```python
from build123d import *

# Parameters (mm, degrees)
F2_DEPTH = 1.778
F3_D     = 3.302
F4_W     = 6.35
F4_H     = 14.4874919379
F4_W_2   = 9.525
F4_W_3   = 11.43
F4_H_2   = 7.62
F4_W_4   = 1.905
F5_DEPTH = 7.62


with BuildPart() as f2:
    # F0 (on Front) → F2 (new body)
    with BuildSketch(Plane.XZ):
        Polygon((-50.8, 24.0124919379), (-50.8, -29.3275080621), (-36.83, -29.3275080621), (0, -29.3275080621), (15.24, -29.3275080621), (15.24, -26.7875080621), (17.235215947, -25.2156577751), (17.235215947, 7.5503422249), (15.24, 9.122192512), (15.24, 20.552192512), (13.716, 24.0124919379), (-35.56, 24.0124919379), align=None)
        with BuildLine():
            ThreePointArc((-35.2425, -26.7875080621), (-35.7074679849, -27.9100400773), (-36.83, -28.3750080621))
            ThreePointArc((-36.83, -28.3750080621), (-37.9525320151, -25.664976047), (-35.2425, -26.7875080621))
        make_face(mode=Mode.SUBTRACT)
        with BuildLine():
            ThreePointArc((-33.9725, 21.4724919379), (-36.6825320151, 20.3499599227), (-35.56, 23.0599919379))
            ThreePointArc((-35.56, 23.0599919379), (-34.4374679849, 22.595023953), (-33.9725, 21.4724919379))
        make_face(mode=Mode.SUBTRACT)
    extrude(amount=F2_DEPTH)

    # F3 (through all)
    with Locations(Plane(origin=(0, 0, 0), x_dir=(1, 0, 0), z_dir=(0, 1, 0))):
        with Locations((15.2230756357, 21.728583892), (15.2230756357, -6.211416108)):
            Hole(F3_D / 2)

    # F4 (on face) → F5 (join)
    with BuildSketch(Plane.XZ.offset(1.778)):
        with Locations((-53.975, 7.2437459689)):
            Rectangle(F4_W, F4_H)
        with Locations((-46.0375, 7.2437459689)):
            Rectangle(F4_W_2, F4_H)
        with Locations((-45.085, -22.3425080621)):
            Rectangle(F4_W_3, F4_H_2)
        with Locations((-51.7525, -22.3425080621)):
            Rectangle(F4_W_4, F4_H_2)
    extrude(amount=F5_DEPTH)


solid = f2.part
```
Check sheet for the modelled part. Datum: model origin and axes. Units: mm. A direction names the side the tool comes from. Round coordinates to 2 decimals unless told otherwise and drop trailing zeros. Write each loop counter-clockwise with the first axis right and the second up, starting at its lowest first coordinate (ties: lowest second). Pieces come first, ordered by that corner, then holes. Notation, with made-up numbers: (23.25, 51.25) -> (47.25, 51.25) arc R27 cw to (47.25, 79.25) -> close; hole circle Ø8 at (42.25, 69.5). An arc over 180 degrees is marked (long way). Put each result on its own line as item: value.
(1) Tool access check on faces 4 (the face through (15.24, -1, -28)), 5 (the face through (-52, -1.778, -22)), 6 (the face through (-49, -6, 0)), 7 (the face through (-41.275, -6, 7)). Record the directions out of +Z, -Z, +X, -X, +Y, -Y that give a thin tool (end or side, any length) a straight path to the whole face; none if there is none.
Values found:
face 4: -Z, +X, +Y, -Y
face 5: +Z, -Z, -X, +Y
face 6: +X, -X, -Y
face 7: +Z, +X, -Y
(2) Sectioned sample at B-B (x = -27). Enter the section's corners in (y, z), plus the area to 3 significant figures.
Values found:
outline: (-1.78, -29.33) -> (0, -29.33) -> (0, 24.01) -> (-1.78, 24.01) -> close
area: 94.8 mm^2
(3) Go/stop test with flat-tipped pins: pin 1 Ø5 at (x, z) = (-53.5, 7.5) entering from +Y; pin 2 Ø2 at (y, z) = (-0.5, -28) entering from +X; pin 3 Ø4 at (x, y) = (-47.5, -7) entering from -Z. Record where each tip stops, or that it passes through.
Values found:
pin 1: stops at y = -1.78
pin 2: stops at x = 15.24
pin 3: stops at z = -26.15
(4) Sectioned sample at C-C (z = 17). Enter the section's corners in (x, y), plus the area to 3 significant figures.
Values found:
outline: (-50.8, -1.78) -> (15.24, -1.78) -> (15.24, 0) -> (-50.8, 0) -> close
area: 117 mm^2
(5) Material ranges on line 1 (Z direction, x = -36.83, y = -1) (1 decimal); line 2 (Z direction, x = -49, y = -5.25); line 3 (Y direction, x = -29, z = 7), recorded low to high.
Values found:
line 1: z = -29.3 to -28.4, -25.2 to 20.5, 22.4 to 24
line 2: z = -26.15 to -18.53, 0 to 14.49
line 3: y = -1.78 to 0
(6) Mould release check, pull along Z, two halves, no side actions. Record for faces 1 (the face through (16.224, -0.877, -26.013)), 2 (the face through (-18, -1, 24.012)), 3 (the face through (15.581, -0.901, -20.117)): released by +Z, released by -Z, zero draft, split by the parting line, or undercut.
Values found:
face 1: released by -Z
face 2: released by +Z
face 3: undercut
